from build123d import *

# Parameters (mm, degrees)
F1_DEPTH = 114.3
F3_DEPTH = 114.3


with BuildPart() as f1:
    # F0 (on Front) → F1 (new body)
    with BuildSketch(Plane.XZ):
        Polygon((0, 12.7), (0, 0), (152.4, 0), (152.4, 12.7), (114.3, 12.7), (114.3, 92.075), (38.1, 92.075), (38.1, 12.7), align=None)
    extrude(amount=F1_DEPTH)

    # F2 (on face) → F3 (cut, through all)
    with BuildSketch(Plane.XZ.offset(114.3)):
        with BuildLine():
            Line((108.393453, 92.075), (45.721143, 92.075))
            ThreePointArc((45.721143, 92.075), (77.057298, 60.801002), (108.393453, 92.075))
        make_face()
    extrude(amount=-F3_DEPTH, mode=Mode.SUBTRACT)


solid = f1.part
Can you work these out from the model? Positions are in its coordinate system, mm. A direction names the side the tool comes from. Coordinates: 2 decimals unless noted, no trailing zeros. Write each loop counter-clockwise with the first axis right and the second up, starting at its lowest first coordinate (ties: lowest second). Pieces come first, ordered by that corner, then holes. Notation, with made-up numbers: (22.25, 40) - (69.25, 40) arc R10 ccw to (69.25, 50) - close; hole circle Ø7 at (52, 48). An arc over 180 degrees is marked (long way). Return JSON: item names as keys, results as strings. Group by question number.
Item 1: If we section it at A-A (z = 71): Write out the boundary of the cut face in (x, y).
Item 2: Which directions (+Z, -Z, +X, -X, +Y, -Y) give clear straight access to the entire face, cutting with the end or side of a thin tool? Please do faces 1 (the face through (42, -56, 92.075)), 2 (the face through (114.3, -56, 52)), 3 (the face through (38.1, -56, 53)).
Item 3: Please list where these lines run through material, in increasing order: probe 1 along Z at (x, y) = (14, -83); probe 2 along X at (y, z) = (-46.5, 22.5); probe 3 along X at (y, z) = (-72, 86).
Item 4: If we section it at B-B (y = -70): Write out the boundary of the cut face in (x, z) (3 decimals).
Item 5: If we section it at D-D (x = 120.5): Write out the boundary of the cut face in (y, z), then the cut area to 3 significant figures.
Item 6: If we section it at C-C (z = 17.5): Write out the boundary of the cut face in (x, y).
Item 7: I'm going to push flat-ended pins straight in: pin 1 Ø10 at (x, y) = (80.5, -74) entering from +Z; pin 2 Ø12 at (y, z) = (-50, 38.5) entering from -X. Where does each tip first touch, or does it pass through?
Return value:
{
 "1": {"outline": "(38.1, -114.3) - (53.92, -114.3) - (53.92, 0) - (38.1, 0) - close; (100.19, -114.3) - (114.3, -114.3) - (114.3, 0) - (100.19, 0) - close"},
 "2": {"face 1": "+Z, +X, -X, +Y, -Y", "face 2": "+Z, +X, +Y, -Y", "face 3": "+Z, -X, +Y, -Y"},
 "3": {"probe 1": "z = 0 to 12.7", "probe 2": "x = 38.1 to 114.3", "probe 3": "x = 38.1 to 46.33, 107.79 to 114.3"},
 "4": {"outline": "(0, 0) - (152.4, 0) - (152.4, 12.7) - (114.3, 12.7) - (114.3, 92.075) - (108.393, 92.075) arc R31.336 cw to (45.721, 92.075) - (38.1, 92.075) - (38.1, 12.7) - (0, 12.7) - close"},
 "5": {"outline": "(-114.3, 0) - (0, 0) - (0, 12.7) - (-114.3, 12.7) - close", "area": "1,450 mm^2"},
 "6": {"outline": "(38.1, -114.3) - (114.3, -114.3) - (114.3, 0) - (38.1, 0) - close"},
 "7": {"pin 1": "stops at z = 61.96", "pin 2": "stops at x = 38.1"}
}
